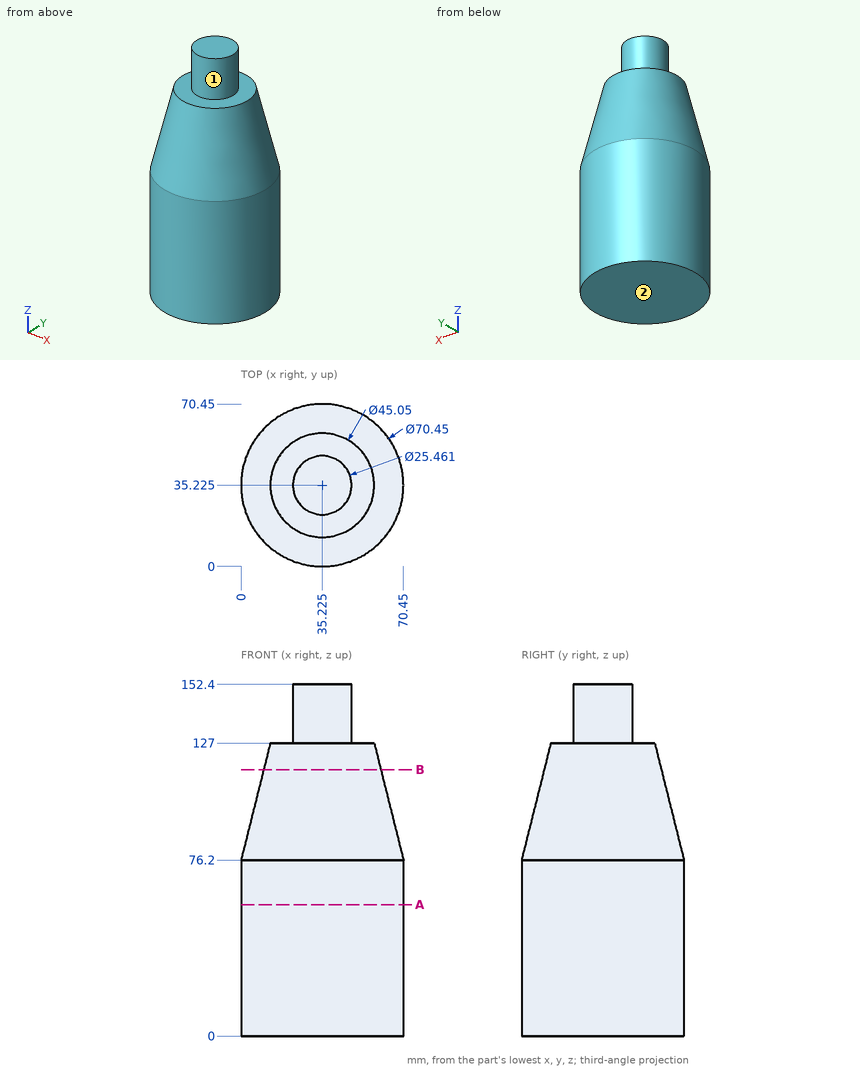
Input: dimensioned drawing with shaded views. Units: mm. Origin: part minimum x, y, z. A direction names the side the tool comes from. Round coordinates to 2 decimals unless told otherwise and drop trailing zeros. Loops run counter-clockwise (first coordinate to the right, second up) from the corner with the lowest first, then second, coordinate; pieces in that order, holes last. Notation, with made-up numbers: M 60,45 L 74,45 A22 cw 74,76 Z; hole C -18,29.25 d7. An arc over 180 degrees is marked long. One line per question, with ' | ' between items.
(1) Contact query for flat-ended pins moving along their axis: P1, Ø3, axis at y = 31, z = 101.5, coming from the -X side; P2, Ø10, axis at x = 53, z = 16, coming from the +Y side; P3, Ø5, axis at x = 13.5, z = 77.5, coming from the +Y side. Output: stop coordinate, or through.
Check result:
P1: stops at x = 6.21 | P2: stops at y = 68.05 | P3: stops at y = 64.51
(2) Cut plane A-A on z = 57. Return the cut outline in (x, y) (3 decimals), plus the area to 3 significant figures.
Check result:
outline: C 35.225,35.225 d70.45 | area: 3,900 mm2
(3) Cut plane B-B on z = 115.5. Return the cut outline in (x, y) (3 decimals), plus the area to 3 significant figures.
Check result:
outline: C 35.225,35.225 d50.8 | area: 2,030 mm2
(4) Access query for the marked faces 1 and 2. Directions: +Z, -Z, +X, -X, +Y, -Y. A direction counts if a zero-diameter tool reaches every point of the face in a straight line with its end or side. Return the directions, or none.
Check result:
face 1: +Z | face 2: -Z, +X, -X, +Y, -Y
(5) Material intervals for line 1 along Z through (x, y) = (18.5, 29); line 2 along Y through (x, z) = (27, 50); line 3 along X through (y, z) = (6.5, 74.5), sorted ascending. Write a range as from..to.
Check result:
line 1: z = 0..127 | line 2: y = 0.97..69.48 | line 3: x = 14.84..55.61
